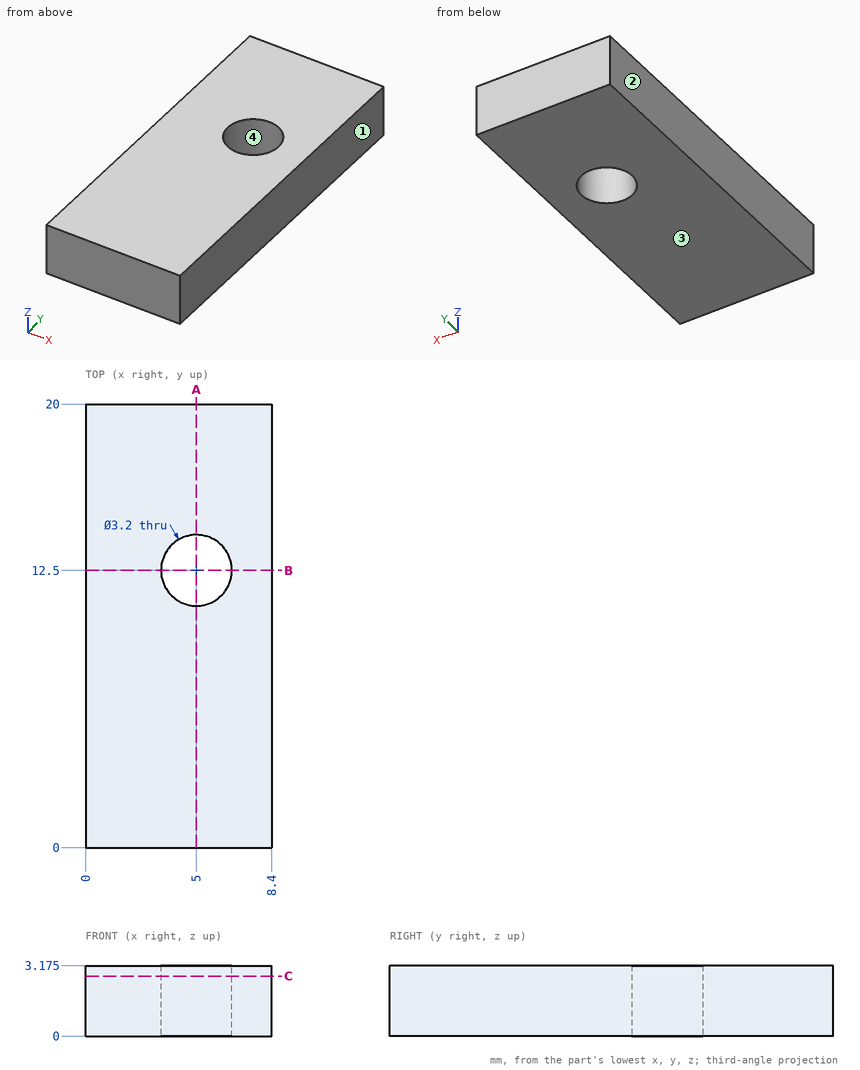
Can you work these out from the drawing? Everything is in mm from the part's minimum corner. Coordinates: 2 decimals unless noted, no trailing zeros. Loops run counter-clockwise (first coordinate to the right, second up) from the corner with the lowest first, then second, coordinate; pieces in that order, holes last. Notation, with made-up numbers: M 77,-38 L 84,-38 A21 ccw 84,-33 Z; hole C 76.25,58.25 d1. An arc over 180 degrees is marked long. One line per item, written item: value.
1. Please list where these lines run through material, in increasing order: probe 1 along Y at (x, z) = (5, 1.5); probe 2 along Y at (x, z) = (4.5, 1.6).
Geometry says:
probe 1: y = 0 to 10.9, 14.1 to 20
probe 2: y = 0 to 10.98, 14.02 to 20
2. Imagine slicing it at A-A (x = 5). List the corners of the cut face in (y, z) for me (3 decimals).
Geometry says:
outline: M 0,0 L 10.9,0 L 10.9,3.175 L 0,3.175 Z; M 14.1,0 L 20,0 L 20,3.175 L 14.1,3.175 Z
3. Imagine slicing it at C-C (z = 2.7). List the corners of the cut face in (x, y) for me, and give its area (3 significant figures).
Geometry says:
outline: M 0,0 L 8.4,0 L 8.4,20 L 0,20 Z; hole C 5,12.5 d3.2
area: 160 mm2
4. Imagine slicing it at B-B (y = 12.5). List the corners of the cut face in (x, z) for me (3 decimals), and give its area (3 significant figures).
Geometry says:
outline: M 0,0 L 3.4,0 L 3.4,3.175 L 0,3.175 Z; M 6.6,0 L 8.4,0 L 8.4,3.175 L 6.6,3.175 Z
area: 16.5 mm2
5. Thinking about a two-plate mould opening in X: for the marked faces 1, 2, 3 and 4, which applies, +X half, -X half, draft (parallel to the pull), parting line (faces both ways), or undercut?
Geometry says:
face 1: +X half
face 2: -X half
face 3: draft
face 4: undercut
